Input: part model. Units: mm. Frame: model coordinates. A direction names the side the tool comes from. Coordinates: 2 decimals unless noted, no trailing zeros. Loops run counter-clockwise (first coordinate to the right, second up) from the corner with the lowest first, then second, coordinate; pieces in that order, holes last. Notation, with made-up numbers: (22.25, 49.5) - (32.25, 49.5) arc R24 cw to (32.25, 65.5) - close; hole circle Ø11 at (21, 31). An arc over 180 degrees is marked (long way). Use one line per item in the form item = value.
from build123d import *

# Parameters (mm, degrees)
CYLINDER065_R     = 1.7
CYLINDER065_DEPTH = 50
CYLINDER066_R     = 1.7
CYLINDER066_DEPTH = 50
CYLINDER063_R     = 2.5
CYLINDER063_DEPTH = 50
CYLINDER064_R     = 4.5
CYLINDER064_DEPTH = 4
BOX039_W          = 20
BOX039_H          = 10
BOX039_DEPTH      = 5


with BuildPart() as m3_studding006:
    # Cylinder065 → Cylinder065 (new body)
    with BuildSketch(Plane(origin=(68.5, 15, 2), x_dir=(1, 0, 0), z_dir=(0, 0, 1))):
        Circle(CYLINDER065_R)
    extrude(amount=CYLINDER065_DEPTH)


with BuildPart() as m3_clearance:
    # Cylinder066 → Cylinder066 (new body)
    with BuildSketch(Plane(origin=(54.5, 15, 2), x_dir=(1, 0, 0), z_dir=(0, 0, 1))):
        Circle(CYLINDER066_R)
    extrude(amount=CYLINDER066_DEPTH)

    # Fusion038: union m3-studding006
    add(m3_studding006.part)


with BuildPart() as nut_clearance:
    # Cylinder063 → Cylinder063 (new body)
    with BuildSketch(Plane(origin=(61.5, 15, 2), x_dir=(1, 0, 0), z_dir=(0, 0, 1))):
        Circle(CYLINDER063_R)
    extrude(amount=CYLINDER063_DEPTH)


with BuildPart() as bearing_nuts001:
    # Cylinder064 → Cylinder064 (new body)
    with BuildSketch(Plane(origin=(61.5, 15, 25), x_dir=(1, 0, 0), z_dir=(0, 0, 1))):
        Circle(CYLINDER064_R)
    extrude(amount=CYLINDER064_DEPTH)

    # Fusion037: union nut-clearance
    add(nut_clearance.part)


with BuildPart() as bearing_cover_b:
    # Box039 → Box039 (new body)
    with BuildSketch(Plane(origin=(51.5, 10, 21), x_dir=(1, 0, 0), z_dir=(0, 0, 1))):
        with Locations((10, 5)):
            Rectangle(BOX039_W, BOX039_H)
    extrude(amount=BOX039_DEPTH)

    # Cut025: cut bearing-nuts001
    add(bearing_nuts001.part, mode=Mode.SUBTRACT)

    # Cut026: cut M3-clearance
    add(m3_clearance.part, mode=Mode.SUBTRACT)


solid = bearing_cover_b.part
Q1. Cut plane D-D, the plane y = 12.75. Return loops of the section in (x, z).
Check values:
outline = (51.5, 21) - (60.41, 21) - (60.41, 25) - (57.6, 25) - (57.6, 26) - (51.5, 26) - close; (62.59, 21) - (71.5, 21) - (71.5, 26) - (65.4, 26) - (65.4, 25) - (62.59, 25) - close
Q2. Cut plane C-C, the plane z = 22.45. Return loops of the section in (x, y).
Check values:
outline = (51.5, 10) - (71.5, 10) - (71.5, 20) - (51.5, 20) - close; hole circle Ø3.4 at (54.5, 15); hole circle Ø5 at (61.5, 15); hole circle Ø3.4 at (68.5, 15)
Q3. Cut plane B-B, the plane y = 15. Return loops of the section in (x, z), then the cut area to 3 significant figures.
Check values:
outline = (51.5, 21) - (52.8, 21) - (52.8, 26) - (51.5, 26) - close; (56.2, 21) - (59, 21) - (59, 25) - (57, 25) - (57, 26) - (56.2, 26) - close; (64, 21) - (66.8, 21) - (66.8, 26) - (66, 26) - (66, 25) - (64, 25) - close; (70.2, 21) - (71.5, 21) - (71.5, 26) - (70.2, 26) - close
area = 37.0 mm²
Q4. Set-up query: faces 4 (the flat face through (51.5, 15, 23)), 5 (the flat face through (63.4, 13.1, 25)). Return all of +Z, -Z, +X, -X, +Y, -Y with unobstructed straight access to the full face (end or side cutting, diameter ignored); none if empty.
Check values:
face_4 = +Z, -Z, -X, +Y, -Y
face_5 = +Z
Q5. First-contact query: P1, Ø4.5, axis at x = 68.5, y = 15, coming from the +Z side. Flat tip, straight axial feed; report the tip coordinate or a pass-through.
Check values:
P1 = 26
Q6. Ray query, line 1 along X through (y, z) = (15, 22.95); line 2 along X through (y, z) = (15, 25.8); line 3 along Y through (x, z) = (54.5, 25). Return the intervals inside material, ascending. Write a range as [from, to].
Check values:
line_1 = [51.5, 52.8], [56.2, 59], [64, 66.8], [70.2, 71.5]
line_2 = [51.5, 52.8], [56.2, 57], [66, 66.8], [70.2, 71.5]
line_3 = [10, 13.3], [16.7, 20]
Q7. Cut plane A-A, the plane x = 61.5. Return loops of the section in (y, z), then the cut area to 3 significant figures.
Check values:
outline = (10, 21) - (12.5, 21) - (12.5, 25) - (10.5, 25) - (10.5, 26) - (10, 26) - close; (17.5, 21) - (20, 21) - (20, 26) - (19.5, 26) - (19.5, 25) - (17.5, 25) - close
area = 21.0 mm²
Q8. Pull-direction query (Y, two-part tool) for faces 1 (the flat face through (61, 20, 23)), 2 (the flat face through (56.9, 16.2, 26)), 3 (the cylindrical face through (66.8, 15.07, 23.46)); classes: pulls with the +Y half, pulls with the -Y half, needs draft (parallel to the pull), parting line crosses it, or undercut.
Check values:
face_1 = pulls with the +Y half
face_2 = needs draft
face_3 = undercut
